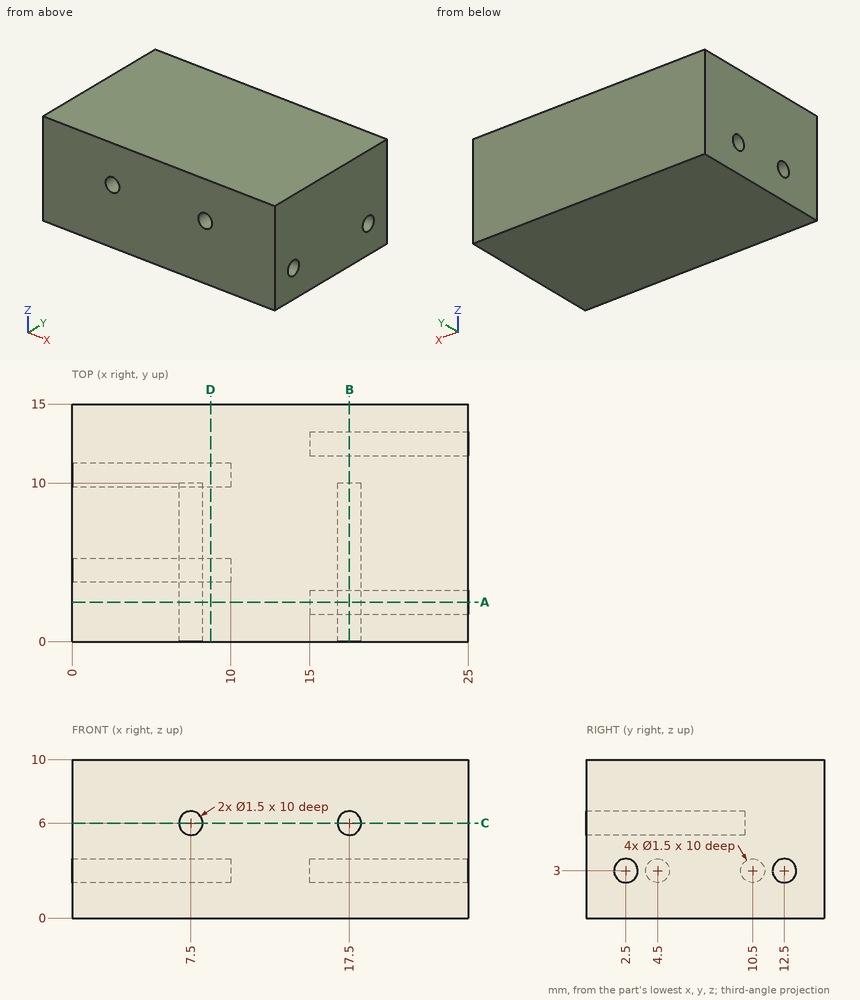
Source: three-view drawing plus pictorial views. Frame: mm from the lowest corner of the part. Round coordinates to 2 decimals unless told otherwise and drop trailing zeros. Write each loop counter-clockwise with the first axis right and the second up, starting at its lowest first coordinate (ties: lowest second). Pieces come first, ordered by that corner, then holes. Notation, with made-up numbers: M -12.5,-0.5 L -8.5,-0.5 A15 cw -8.5,6.5 Z; hole C -14.75,70 d10. An arc over 180 degrees is marked long. One line per item, written item: value. Start each with the question number.
Item 1: Section query D-D (x = 8.75). Return the cut outline in (y, z), plus the area to 3 significant figures.
Item 2: Section query C-C (z = 6). Return the cut outline in (x, y), plus the area to 3 significant figures.
Item 3: Section query A-A (y = 2.5). Return the cut outline in (x, z), plus the area to 3 significant figures.
Item 4: Pin query (flat end, axial travel): pin 1 (0.8 mm diameter, centred on x = 17.5, z = 6, fed in from -Y); pin 2 (0.9 mm diameter, centred on y = 4.5, z = 3, fed in from -X); pin 3 (1.2 mm diameter, centred on y = 2.5, z = 3, fed in from +X). Return the tip coordinate at first contact, or that it passes through.
Item 5: Section query B-B (x = 17.5). Return the cut outline in (y, z).
Item 6: Ray query, L1, parallel to Y at x = 20.75, z = 3; L2, parallel to Z at x = 17.5, y = 8.25; L3, parallel to Y at x = 7.25, z = 2.5. Return the intervals inside material, ascending. Write a range as from..to.
Result set:
1. outline: M 0,0 L 15,0 L 15,10 L 0,10 Z; hole C 4.5,3 d1.5; hole C 10.5,3 d1.5
1. area: 146 mm²
2. outline: M 0,0 L 6.75,0 L 6.75,10 L 8.25,10 L 8.25,0 L 16.75,0 L 16.75,10 L 18.25,10 L 18.25,0 L 25,0 L 25,15 L 0,15 Z
2. area: 345 mm²
3. outline: M 0,0 L 25,0 L 25,2.25 L 15,2.25 L 15,3.75 L 25,3.75 L 25,10 L 0,10 Z; hole C 7.5,6 d1.5; hole C 17.5,6 d1.5
3. area: 231 mm²
4. pin 1: stops at y = 10
4. pin 2: stops at x = 10
4. pin 3: stops at x = 15
5. outline: M 0,0 L 15,0 L 15,10 L 0,10 L 0,6.75 L 10,6.75 L 10,5.25 L 0,5.25 Z; hole C 2.5,3 d1.5; hole C 12.5,3 d1.5
6. L1: y = 0..1.75, 3.25..11.75, 13.25..15
6. L2: z = 0..5.25, 6.75..10
6. L3: y = 0..3.94, 5.06..9.94, 11.06..15
